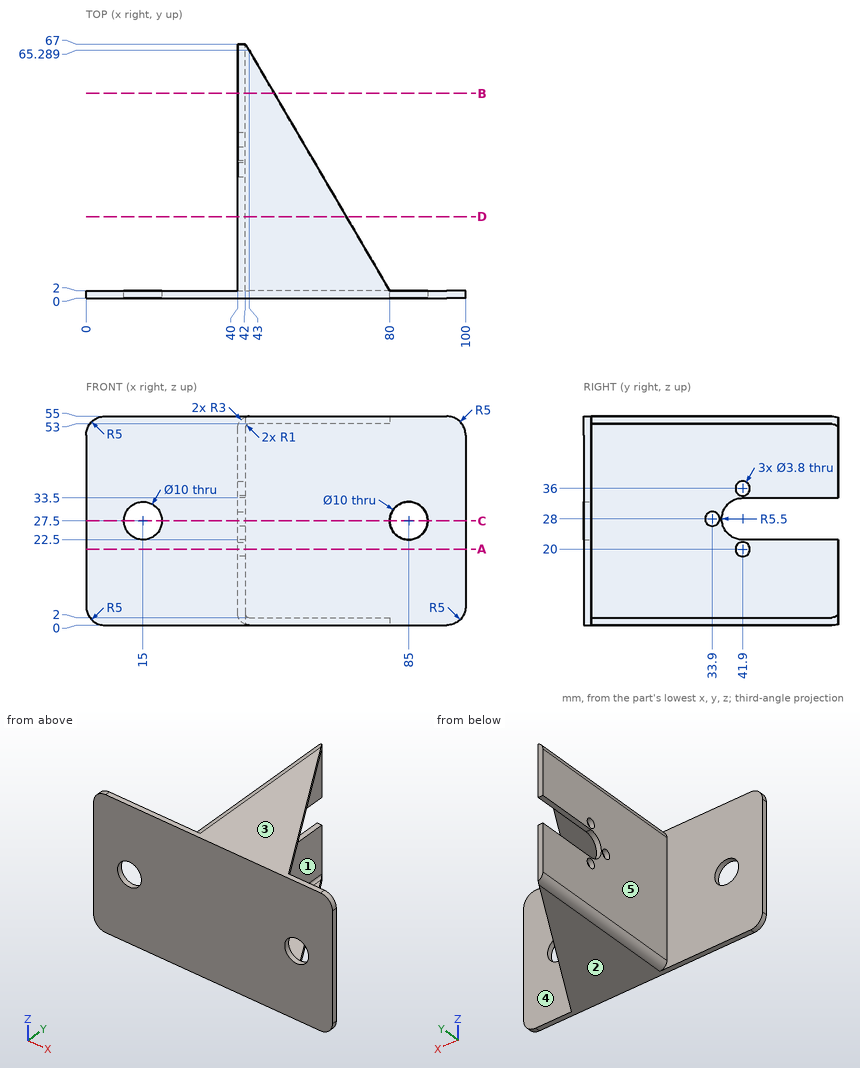
The figure shows three views and two pictorial views of one solid part (mm, origin at its lowest corner). Answer the questions. A direction names the side the tool comes from. Give positions to 0.01 mm unless a question says otherwise; leave off trailing zeros. Order: outer loops, then holes, each group sorted by start corner. A loop starts at its lowest first (then second) coordinate and runs counter-clockwise, first axis right, second up. Notation, with made-up numbers: (86, 60) -> (145, 60) arc R21 ccw to (145, 92) -> close; hole circle Ø2 at (82.5, 11.25). An arc over 180 degrees is marked (long way). Write each question's results on one line, items separated by ' | '.
Q1. Straight lines are drawn through the part: probe 1 along X at (y, z) = (1, 27) (1 decimal); probe 2 along Y at (x, z) = (40.5, 28); probe 3 along Y at (x, z) = (40.9, 36). For each, find the intervals that lie inside material, in ascending order. Write a range as from..to.
Checked values:
probe 1: x = 0..10, 20..80, 90..100 | probe 2: y = 0..32, 35.8..36.4 | probe 3: y = 0..40, 43.8..67
Q2. The part is cut by section D-D, the plane y = 21.5. Give the vertices of the cut face in (x, z).
Checked values:
outline: (40, 3) arc R3 ccw to (43, 0) -> (68.6, 0) -> (68.6, 2) -> (43, 2) arc R1 cw to (42, 3) -> (42, 52) arc R1 cw to (43, 53) -> (68.6, 53) -> (68.6, 55) -> (43, 55) arc R3 ccw to (40, 52) -> close
Q3. The part is cut by section A-A, the plane z = 20. Give the vertices of the cut face in (x, y).
Checked values:
outline: (0, 0) -> (100, 0) -> (100, 2) -> (42, 2) -> (42, 40) -> (40, 40) -> (40, 2) -> (0, 2) -> close; (40, 43.8) -> (42, 43.8) -> (42, 67) -> (40, 67) -> close
Q4. Determine the mould class of the marked faces 3, 4 and 5 for opening direction Z: pulls with the +Z half, pulls with the -Z half, needs draft (parallel to the pull), parting line crosses it, or undercut.
Checked values:
face 3: pulls with the +Z half | face 4: undercut | face 5: needs draft
Q5. The part is cut by section C-C, the plane z = 27.5. Give the vertices of the cut face in (x, y).
Checked values:
outline: (0, 0) -> (10, 0) -> (10, 2) -> (0, 2) -> close; (20, 0) -> (80, 0) -> (80, 2) -> (42, 2) -> (42, 32.07) -> (40, 32.07) -> (40, 2) -> (20, 2) -> close; (40, 35.73) -> (42, 35.73) -> (42, 36.42) -> (40, 36.42) -> close; (90, 0) -> (100, 0) -> (100, 2) -> (90, 2) -> close
Q6. The part is cut by section B-B, the plane y = 54. Give the vertices of the cut face in (x, z), and give its area (3 significant figures).
Checked values:
outline: (40, 3) arc R3 ccw to (43, 0) -> (49.6, 0) -> (49.6, 2) -> (43, 2) arc R1 cw to (42, 3) -> (42, 22.5) -> (40, 22.5) -> close; (40, 33.5) -> (42, 33.5) -> (42, 52) arc R1 cw to (43, 53) -> (49.6, 53) -> (49.6, 55) -> (43, 55) arc R3 ccw to (40, 52) -> close | area: 115 mm^2
Q7. Each of these flat-tipped pins is pushed along its axis until it touches: P1, Ø1.5, axis at y = 41.5, z = 6, coming from the +X side; P2, Ø8, axis at x = 31.5, z = 33.5, coming from the +Y side; P3, Ø14.5, axis at y = 28.5, z = 22, coming from the -X side. Where does it stop, or does it pass through?
Checked values:
P1: stops at x = 42 | P2: stops at y = 2 | P3: stops at x = 40
Q8. Which of the six approach directions +Z, -Z, +X, -X, +Y, -Y give full straight-line access (tool end or side, diameter ignored) to the marked faces 1 and 2?
Checked values:
face 1: +X, +Y | face 2: -Z, +X, -X, +Y, -Y
